```python
from build123d import *

# Parameters (mm, degrees)
SKETCH3_W           = 104
SKETCH3_H           = 94
SKETCH3_W_2         = 100
SKETCH3_H_2         = 90
EXTRUDE_THIN1_DEPTH = 86
SKETCH3_2_W         = 100
SKETCH3_2_H         = 90
BOSS_EXTRUDE1_DEPTH = 2
SKETCH6_W           = 104
SKETCH6_H           = 94
SKETCH6_W_2         = 73.912331144
SKETCH6_H_2         = 63.926876015
BOSS_EXTRUDE2_DEPTH = 2
LPATTERN1_COUNT     = 2
LPATTERN1_PITCH     = 40
LPATTERN2_COUNT     = 2
LPATTERN2_PITCH     = 60
CUT_EXTRUDE1_REACH  = 134.868
SKETCH9_R           = 1.5
SKETCH10_W          = 18
SKETCH10_H          = 40
BOSS_EXTRUDE3_DEPTH = 8.5
SKETCH12_W          = 35
SKETCH12_H          = 6
CUT_EXTRUDE2_DEPTH  = 65.5


with BuildPart() as part:
    # Sketch3 → Extrude-Thin1 (new body)
    with BuildSketch(Plane.XY):
        with Locations((18.667779633, -23.113522538)):
            Rectangle(SKETCH3_W, SKETCH3_H)
        with Locations((18.667779633, -23.113522538)):
            Rectangle(SKETCH3_W_2, SKETCH3_H_2, mode=Mode.SUBTRACT)
    extrude(amount=EXTRUDE_THIN1_DEPTH)

    # Sketch3<2> → Boss-Extrude1 (add)
    with BuildSketch(Plane.XY):
        with Locations((18.667779633, -23.113522538)):
            Rectangle(SKETCH3_2_W, SKETCH3_2_H)
    extrude(amount=BOSS_EXTRUDE1_DEPTH)

    # Sketch6 → Boss-Extrude2 (add)
    with BuildSketch(Plane.XY.offset(86)):
        with Locations((18.667779633, -23.113522538)):
            Rectangle(SKETCH6_W, SKETCH6_H)
        with Locations((18.623945205, -23.076960546)):
            Rectangle(SKETCH6_W_2, SKETCH6_H_2, mode=Mode.SUBTRACT)
    boss_extrude2 = extrude(amount=BOSS_EXTRUDE2_DEPTH)

    # LPattern1: Boss-Extrude2 ×2
    with Locations(*[(0, 0, -i * LPATTERN1_PITCH) for i in range(1, LPATTERN1_COUNT)]):
        add(boss_extrude2)

    # LPattern2: Boss-Extrude2 ×2
    with Locations(*[(0, 0, -i * LPATTERN2_PITCH) for i in range(1, LPATTERN2_COUNT)]):
        add(boss_extrude2)

    # Cut-Extrude1: up to this face of the body (flat: up to its plane)
    cut_extrude1_end = Plane(part.part.faces().sort_by_distance((18.667779633, -23.113522538, 2))[0])
    # Sketch9 → Cut-Extrude1 (cut, up to the picked face)
    with BuildSketch(Plane.XY.offset(88), mode=Mode.PRIVATE) as cut_extrude1_sk1:
        with Locations((-25.492242635, 15.664652421)):
            Circle(SKETCH9_R)
    cut_extrude1_tool1 = split(extrude(cut_extrude1_sk1.sketch, amount=-CUT_EXTRUDE1_REACH, mode=Mode.PRIVATE), bisect_by=cut_extrude1_end, keep=Keep.BOTH, mode=Mode.PRIVATE)
    # Sketch9 → Cut-Extrude1 (cut, up to the picked face)
    with BuildSketch(Plane.XY.offset(88), mode=Mode.PRIVATE) as cut_extrude1_sk2:
        with Locations((38.007757365, 15.664652421)):
            Circle(SKETCH9_R)
    cut_extrude1_tool2 = split(extrude(cut_extrude1_sk2.sketch, amount=-CUT_EXTRUDE1_REACH, mode=Mode.PRIVATE), bisect_by=cut_extrude1_end, keep=Keep.BOTH, mode=Mode.PRIVATE)
    # Sketch9 → Cut-Extrude1 (cut, up to the picked face)
    with BuildSketch(Plane.XY.offset(88), mode=Mode.PRIVATE) as cut_extrude1_sk3:
        with Locations((38.007757365, -22.435347579)):
            Circle(SKETCH9_R)
    cut_extrude1_tool3 = split(extrude(cut_extrude1_sk3.sketch, amount=-CUT_EXTRUDE1_REACH, mode=Mode.PRIVATE), bisect_by=cut_extrude1_end, keep=Keep.BOTH, mode=Mode.PRIVATE)
    # Sketch9 → Cut-Extrude1 (cut, up to the picked face)
    with BuildSketch(Plane.XY.offset(88), mode=Mode.PRIVATE) as cut_extrude1_sk4:
        with Locations((38.007757365, -60.535347579)):
            Circle(SKETCH9_R)
    cut_extrude1_tool4 = split(extrude(cut_extrude1_sk4.sketch, amount=-CUT_EXTRUDE1_REACH, mode=Mode.PRIVATE), bisect_by=cut_extrude1_end, keep=Keep.BOTH, mode=Mode.PRIVATE)
    # Sketch9 → Cut-Extrude1 (cut, up to the picked face)
    with BuildSketch(Plane.XY.offset(88), mode=Mode.PRIVATE) as cut_extrude1_sk5:
        with Locations((-25.492242635, -22.435347579)):
            Circle(SKETCH9_R)
    cut_extrude1_tool5 = split(extrude(cut_extrude1_sk5.sketch, amount=-CUT_EXTRUDE1_REACH, mode=Mode.PRIVATE), bisect_by=cut_extrude1_end, keep=Keep.BOTH, mode=Mode.PRIVATE)
    # Sketch9 → Cut-Extrude1 (cut, up to the picked face)
    with BuildSketch(Plane.XY.offset(88), mode=Mode.PRIVATE) as cut_extrude1_sk6:
        with Locations((-25.492242635, -60.535347579)):
            Circle(SKETCH9_R)
    cut_extrude1_tool6 = split(extrude(cut_extrude1_sk6.sketch, amount=-CUT_EXTRUDE1_REACH, mode=Mode.PRIVATE), bisect_by=cut_extrude1_end, keep=Keep.BOTH, mode=Mode.PRIVATE)
    add(cut_extrude1_tool1.solids().sort_by(Axis((-25.492243, 15.664652, 88), (0, 0, -1)))[0], mode=Mode.SUBTRACT)
    add(cut_extrude1_tool2.solids().sort_by(Axis((38.007757, 15.664652, 88), (0, 0, -1)))[0], mode=Mode.SUBTRACT)
    add(cut_extrude1_tool3.solids().sort_by(Axis((38.007757, -22.435348, 88), (0, 0, -1)))[0], mode=Mode.SUBTRACT)
    add(cut_extrude1_tool4.solids().sort_by(Axis((38.007757, -60.535348, 88), (0, 0, -1)))[0], mode=Mode.SUBTRACT)
    add(cut_extrude1_tool5.solids().sort_by(Axis((-25.492243, -22.435348, 88), (0, 0, -1)))[0], mode=Mode.SUBTRACT)
    add(cut_extrude1_tool6.solids().sort_by(Axis((-25.492243, -60.535348, 88), (0, 0, -1)))[0], mode=Mode.SUBTRACT)

    # Sketch10 → Boss-Extrude3 (add)
    with BuildSketch(Plane.XZ.offset(70.113522538)):
        with Locations((-5.791529817, 49.453628138)):
            Rectangle(SKETCH10_W, SKETCH10_H)
        with Locations((39.794952927, 49.453628138)):
            Rectangle(SKETCH10_W, SKETCH10_H)
    extrude(amount=BOSS_EXTRUDE3_DEPTH)

    # Sketch12 → Cut-Extrude2 (cut)
    with BuildSketch(Plane(origin=(48.794952927, 0, 0), x_dir=(0, 0, -1), z_dir=(1, 0, 0))):
        with Locations((-49.453628138, -73.113522538)):
            Rectangle(SKETCH12_W, SKETCH12_H)
    extrude(amount=-CUT_EXTRUDE2_DEPTH, mode=Mode.SUBTRACT)


solid = part.part
```
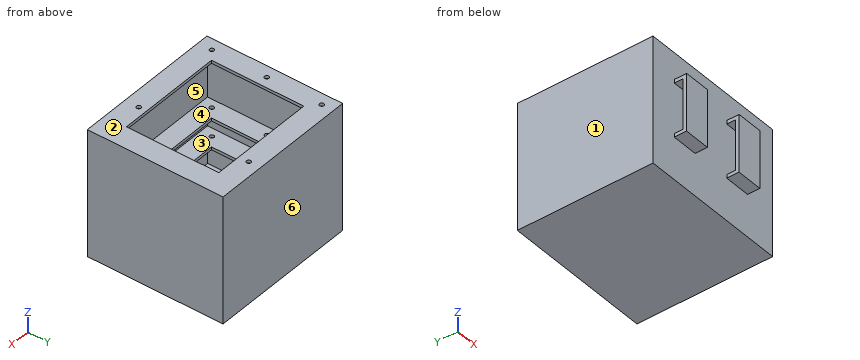
Check sheet for the modelled part. Datum: model origin and axes. Units: mm. Face numbers are marked on the shaded views. A direction names the side the tool comes from. Coordinates: 2 decimals unless noted, no trailing zeros. Loops run counter-clockwise (first coordinate to the right, second up) from the corner with the lowest first, then second, coordinate; pieces in that order, holes last. Notation, with made-up numbers: M -23,57 L 7,57 A26 ccw 7,96 Z; hole C 21,9.25 d10. An arc over 180 degrees is marked long. Answer as a JSON object with one key per item and string values.
1. Sectioned sample at B-B on x = 9.5. Record the cut outline in (y, z), and give its area (3 significant figures).
Outcome:
{"outline": "M -70.11,0 L 23.89,0 L 23.89,88 L 8.89,88 L 8.89,86 L 21.89,86 L 21.89,48 L 8.89,48 L 8.89,46 L 21.89,46 L 21.89,28 L 8.89,28 L 8.89,26 L 21.89,26 L 21.89,2 L -68.11,2 L -68.11,26 L -55.04,26 L -55.04,28 L -68.11,28 L -68.11,46 L -55.04,46 L -55.04,48 L -68.11,48 L -68.11,86 L -55.04,86 L -55.04,88 L -70.11,88 Z", "area": "688 mm²"}
2. Sectioned sample at C-C on z = 79. Record the cut outline in (x, y).
Outcome:
{"outline": "M -33.33,-70.11 L 70.67,-70.11 L 70.67,23.89 L -33.33,23.89 Z; hole M -31.33,-68.11 L 68.67,-68.11 L 68.67,21.89 L -31.33,21.89 Z"}
3. Sectioned sample at D-D on y = 5. Record the cut outline in (x, z).
Outcome:
{"outline": "M -33.33,0 L 70.67,0 L 70.67,88 L 55.58,88 L 55.58,86 L 68.67,86 L 68.67,48 L 55.58,48 L 55.58,46 L 68.67,46 L 68.67,28 L 55.58,28 L 55.58,26 L 68.67,26 L 68.67,2 L -31.33,2 L -31.33,26 L -18.33,26 L -18.33,28 L -31.33,28 L -31.33,46 L -18.33,46 L -18.33,48 L -31.33,48 L -31.33,86 L -18.33,86 L -18.33,88 L -33.33,88 Z"}
4. Depth check by flat-ended pin: P1, Ø2.5, axis at x = 39.5, y = -76, coming from the -Z side; P2, Ø2, axis at x = 37, z = 87, coming from the -Y side; P3, Ø2.5, axis at y = -75, z = 55.5, coming from the -X side. Enter the tip coordinate at first touch or a pass-through.
Outcome:
{"P1": "z = 29.45", "P2": "y = -70.11", "P3": "x = -14.79"}
5. Access from +Z, -Z, +X, -X, +Y, -Y to the whole of each face (thin tool, end or side, straight path). Record for the marked faces 5 and 6.
Outcome:
{"face 5": "none", "face 6": "+Z, -Z, +X, -X, +Y"}
6. Scan lines: L1, parallel to Z at x = 31.5, y = -62.5; L2, parallel to Y at x = 0, z = 62; L3, parallel to Y at x = 64.5, z = 11.5. Record each from-to range of solid material in increasing order. Write a range as from..to.
Outcome:
{"L1": "0..2, 26..28, 46..48, 86..88", "L2": "-78.61..-76.11, -70.11..-68.11, 21.89..23.89", "L3": "-70.11..-68.11, 21.89..23.89"}
7. Release check for a two-part mould opening along Z. For the marked faces 1, 2, 3 and 4 record: pulls with the +Z half, pulls with the -Z half, needs draft (parallel to the pull), parting line crosses it, or undercut.
Outcome:
{"face 1": "needs draft", "face 2": "pulls with the +Z half", "face 3": "undercut", "face 4": "undercut"}
8. Sectioned sample at A-A on z = 36. Record the cut outline in (x, y).
Outcome:
{"outline": "M -33.33,-70.11 L 70.67,-70.11 L 70.67,23.89 L -33.33,23.89 Z; M -14.79,-78.61 L 3.21,-78.61 L 3.21,-76.11 L -14.79,-76.11 Z; M 30.79,-78.61 L 48.79,-78.61 L 48.79,-76.11 L 30.79,-76.11 Z; hole M -31.33,-68.11 L 68.67,-68.11 L 68.67,21.89 L -31.33,21.89 Z"}
